```python
from build123d import *

# Parameters (mm, degrees)
F1_DEPTH      = 10
F2_R          = 14
F3_DEPTH      = 25
F3_DEPTH_BACK = 25
F5_START      = 1
F4_R          = 14.25
F5_DEPTH      = 8
F6_R          = 1
F7_R          = 1


with BuildPart() as f1:
    # F0 (on Top) → F1 (new body)
    with BuildSketch(Plane.XY):
        with BuildLine():
            ThreePointArc((17.9071800695, -15.3580631832), (30.1934118694, -11.6766585315), (35.5, 0))
            ThreePointArc((35.5, 0), (30.1934118694, 11.6766585315), (17.9071800695, 15.3580631832))
            ThreePointArc((17.9071800695, 15.3580631832), (4.5, 0), (17.9071800695, -15.3580631832))
        make_face()
        with BuildLine():
            ThreePointArc((5.5, 17.3205080757), (5.2089888633, 20.3099323942), (4.3468828701, 23.1871043555))
            ThreePointArc((4.3468828701, 23.1871043555), (-17.7499998668, 30.7439019112), (-22.2540630355, 7.8290414281))
            ThreePointArc((-22.2540630355, 7.8290414281), (-4.9844231164, 2.6544251452), (5.5, 17.3205080757))
        make_face()
        with BuildLine():
            ThreePointArc((-22.2540628496, -7.8290411881), (-17.7500000176, -30.7439018242), (4.3468828532, -23.1871043968))
            ThreePointArc((4.3468828532, -23.1871043968), (5.208988859, -20.3099324162), (5.5, -17.3205080757))
            ThreePointArc((5.5, -17.3205080757), (-4.9844229728, -2.6544251943), (-22.2540628496, -7.8290411881))
        make_face()
        with BuildLine():
            ThreePointArc((17.9071800695, -15.3580631832), (4.5, 0), (17.9071800695, 15.3580631832))
            ThreePointArc((17.9071800695, 15.3580631832), (9.7883250707, 16.9538762501), (4.3468828701, 23.1871043555))
            ThreePointArc((4.3468828701, 23.1871043555), (5.2089888633, 20.3099323942), (5.5, 17.3205080757))
            ThreePointArc((5.5, 17.3205080757), (-4.9844231164, 2.6544251452), (-22.2540630355, 7.8290414281))
            ThreePointArc((-22.2540630355, 7.8290414281), (-20.264507037, 4.1371013379), (-19.5766500605, 0))
            ThreePointArc((-19.5766500605, 0), (-20.2645069879, -4.1371011943), (-22.2540628496, -7.8290411881))
            ThreePointArc((-22.2540628496, -7.8290411881), (-4.9844229728, -2.6544251943), (5.5, -17.3205080757))
            ThreePointArc((5.5, -17.3205080757), (5.208988859, -20.3099324162), (4.3468828532, -23.1871043968))
            ThreePointArc((4.3468828532, -23.1871043968), (9.7883250513, -16.9538762612), (17.9071800695, -15.3580631832))
        make_face()
    extrude(amount=F1_DEPTH)

    # F2 (on Top) → F3 (cut, two sides)
    with BuildSketch(Plane.XY) as f3_sk:
        with Locations((20, 0)):
            Circle(F2_R)
        with Locations((-10, 17.3205080757)):
            Circle(F2_R)
        with Locations((-10, -17.3205080757)):
            Circle(F2_R)
    extrude(amount=-F3_DEPTH, mode=Mode.SUBTRACT)
    extrude(f3_sk.sketch, amount=F3_DEPTH_BACK, mode=Mode.SUBTRACT)

    # F4 (on Top) → F5 (cut)
    with BuildSketch(Plane.XY.offset(F5_START)):
        with Locations((20, 0)):
            Circle(F4_R)
        with Locations((-10, 17.3205080757)):
            Circle(F4_R)
        with Locations((-10, -17.3205080757)):
            Circle(F4_R)
    extrude(amount=F5_DEPTH, mode=Mode.SUBTRACT)

    # F6
    f6_edges = [f1.edges().sort_by_distance(p)[0] for p in [
        (-17.75, -30.743902, 10),
        (9.788325, -16.953876, 10),
        (35.5, 0, 10),
        (9.788325, 16.953876, 10),
        (-19.57665, 0, 10),
        (-17.75, 30.743902, 10),
    ]]
    fillet(f6_edges, radius=F6_R)

    # F7
    f7_edges = [f1.edges().sort_by_distance(p)[0] for p in [
        (-17.75, 30.743902, 0),
        (9.788325, 16.953876, 0),
        (35.5, 0, 0),
        (9.788325, -16.953876, 0),
        (-17.75, -30.743902, 0),
        (-19.57665, 0, 0),
    ]]
    fillet(f7_edges, radius=F7_R)


solid = f1.part
```
Source: CAD feature listing. Evaluate the final solid. Frame: model axes, mm. A direction names the side the tool comes from. Coordinates: 2 decimals unless noted, no trailing zeros. Loops run counter-clockwise (first coordinate to the right, second up) from the corner with the lowest first, then second, coordinate; pieces in that order, holes last. Notation, with made-up numbers: M 7,55 L 48,55 A18 cw 48,73 Z; hole C 57.5,57 d2. An arc over 180 degrees is marked long. Use CSV: the item, a comma, the result in double quotes.
(1) Draft query along Y for faces 1 (the face through (9.891, 16.895, 4.944)), 2 (the face through (9.69, -17.01, 4.94)), 3 (the face through (3.354, 21.526, 9.493)), 4 (the face through (33.35, 4.21, 0.49)). Return one class per face: pulls with the +Y half, pulls with the -Y half, needs draft (parallel to the pull), parting line crosses it, or undercut.
Answers follow:
face 1,"pulls with the +Y half"
face 2,"pulls with the -Y half"
face 3,"undercut"
face 4,"undercut"
(2) Cut plane A-A on z = 6. Return loops of the section in (x, y).
Answers follow:
outline,"M -22.25,-7.83 A15.5 ccw long 4.35,-23.19 A12.79 cw 17.91,-15.36 A15.5 ccw long 17.91,15.36 A12.79 cw 4.35,23.19 A15.5 ccw long -22.25,7.83 A12.79 cw Z; hole C -10,-17.32 d28.5; hole C -10,17.32 d28.5; hole C 20,0 d28.5"
(3) Contact query for flat-ended pins moving along their axis: pin 1 (23 mm diameter, centred on x = -10, y = 24.5, fed in from +Z); pin 2 (1.5 mm diameter, centred on x = -15, z = 8, fed in from +Y); pin 3 (1.5 mm diameter, centred on y = -10, z = 4.5, fed in from -X); pin 4 (6 mm diameter, centred on y = 4, z = 3, fed in from -X). Output: stop coordinate, or through.
Answers follow:
pin 1,"z = 10"
pin 2,"y = 32.23"
pin 3,"x = -24.04"
pin 4,"x = -21.66"
(4) Line query: line 1 (Y direction, x = -10, z = 3.25); line 2 (X direction, y = 9.5, z = 3); line 3 (X direction, y = 11.5, z = 8.25). Output: solid intervals per line, ascending. Write a range as [from, to].
Answers follow:
line 1,"[-32.82, -31.57], [-3.07, 3.07], [31.57, 32.82]"
line 2,"[-23.38, -21.91], [1.91, 9.38], [30.62, 32.25]"
line 3,"[-24.37, -23.01], [3.01, 11.58], [28.42, 30.39]"
(5) Reachability of faces 5 (the face through (-17.427, 30.925, 4.944)), 6 (the face through (3.59, -13.04, 4.94)) from +Z, -Z, +X, -X, +Y, -Y: full face, straight path, thin tool, end or side. Return the list, or none.
Answers follow:
face 5,"+Z, -Z"
face 6,"none"
(6) Cut plane B-B on x = -10. Give the number of separate pieces and of enclosed holes in the cut face, and give its area (3 significant figures).
Answers follow:
separate pieces,"3"
enclosed holes,"0"
area,"87.6 mm²"
